Input: part model. Units: mm. Frame: model coordinates. Face numbers are marked on the shaded views. Give positions to 0.01 mm unless a question says otherwise; leave off trailing zeros. Order: outer loops, then holes, each group sorted by start corner. A loop starts at its lowest first (then second) coordinate and runs counter-clockwise, first axis right, second up. Notation, with made-up numbers: (54.25, 81) -> (76.25, 81) arc R29 cw to (76.25, 103) -> close; hole circle Ø1 at (38, 19). An arc over 180 degrees is marked (long way). Use a Markdown table: item, result. Add a question column.
Autodesk Inventor part; units mm, degrees
ref_plane "YZ Plane" through (0, 0, 0) normal (1, 0, 0) x (0, 1, 0)
ref_plane "XZ Plane" through (0, 0, 0) normal (0, 1, 0) x (-1, 0, 0)
ref_plane "XY Plane" through (0, 0, 0) normal (0, 0, 1) x (1, 0, 0)
sketch "Skizze2" plane through (0, 0, 0) normal (0, 0, 1) x (1, 0, 0)
  line L0 (-26.1954, 0) -> (26.1954, 0)
  line L1 (0, -30.2532) -> (0, 68.0422)
  line L2 (-18.5, 54) -> (-18.5, -6.7574)
  line L3 (-9.2574, -16) -> (9.2574, -16)
  line L4 (18.5, -6.7574) -> (18.5, 54)
  line L5 (18.5, 54) -> (11, 54)
  line L6 (11, 54) -> (11, 4.2426)
  line L7 (-11, 4.2426) -> (-11, 54)
  line L8 (-11, 54) -> (-18.5, 54)
  circle A0 centre (0, -10) radius 3.15
  circle A1 centre (-14.75, 43) radius 1.15
  circle A2 centre (-14.75, 30) radius 1.15
  circle A3 centre (-14.75, 17) radius 1.15
  circle A4 centre (-14.75, 3) radius 1.15
  circle A5 centre (14.75, 43) radius 1.15
  circle A6 centre (14.75, 30) radius 1.15
  circle A7 centre (14.75, 17) radius 1.15
  circle A8 centre (14.75, 3) radius 1.15
  line L9 (-17.6213, -8.8787) -> (-11.3787, -15.1213)
  line L10 (11.3787, -15.1213) -> (17.6213, -8.8787)
  arc A9 (-18.5, -6.7574) -> (-17.6213, -8.8787) centre (-15.5, -6.7574) ccw
  arc A10 (-11.3787, -15.1213) -> (-9.2574, -16) centre (-9.2574, -13) ccw
  arc A11 (9.2574, -16) -> (11.3787, -15.1213) centre (9.2574, -13) ccw
  line L11 (-11, 4.2426) -> (-11, 1.4853)
  line L12 (11, 4.2426) -> (11, 1.4853)
  line L13 (-6.7574, -2.7574) -> (6.7574, -2.7574)
  line L14 (-10.1213, -0.636) -> (-8.8787, -1.8787)
  line L15 (8.8787, -1.8787) -> (10.1213, -0.636)
  arc A12 (-11, 1.4853) -> (-10.1213, -0.636) centre (-8, 1.4853) ccw
  arc A13 (-8.8787, -1.8787) -> (-6.7574, -2.7574) centre (-6.7574, 0.2426) ccw
  arc A14 (6.7574, -2.7574) -> (8.8787, -1.8787) centre (6.7574, 0.2426) ccw
  arc A15 (10.1213, -0.636) -> (11, 1.4853) centre (8, 1.4853) ccw
  arc A16 (17.6213, -8.8787) -> (18.5, -6.7574) centre (15.5, -6.7574) ccw
  point P0 (0, 0)
  point P1 (-18.5, -16)
  point P2 (18.5, -16)
  point P3 (11, 0)
  point P4 (-11, 0)
  point P5 (-8, 0)
  point P6 (-11, 3)
  point P7 (8, 0)
  point P8 (11, 3)
  point P9 (-18.5, -8)
  point P10 (-10.5, -16)
  point P11 (10.5, -16)
  point P12 (18.5, -8)
  point P13 (-11, -2.7574)
  point P14 (11, -2.7574)
  point P15 (-11, 0.2426)
  point P16 (-8, -2.7574)
  point P17 (8, -2.7574)
  point P18 (11, 0.2426)
  dimension "d0" = 70
  dimension "d1" = 37
  dimension "d2" = 90
  dimension "d3" = 70
  dimension "d4" = 90
  dimension "d6" = 7.5
  dimension "d8" = 90
  dimension "d9" = 22
  dimension "d10" = 54
  dimension "d11" = 6.3
  dimension "d13" = 6
  dimension "d14" = 2.3
  dimension "d15" = 3.75
  dimension "d16" = 11
  dimension "d17" = 2.3
  dimension "d18" = 2.3
  dimension "d19" = 2.3
  dimension "d20" = 13
  dimension "d21" = 13
  dimension "d22" = 14
  dimension "d23" = 3.75
  dimension "d24" = 3.75
  dimension "d25" = 3.75
  dimension "d26" = 2.3
  dimension "d27" = 2.3
  dimension "d28" = 2.3
  dimension "d29" = 2.3
  dimension "d30" = 3.75
  dimension "d31" = 3
  dimension "d32" = 3
  dimension "d33" = 3
  dimension "d34" = 3
  dimension "d35" = 8
  dimension "d36" = 8
  dimension "d37" = 8
  dimension "d38" = 8
  dimension "d45" = 7
  dimension "d46" = 7
  dimension "d47" = 3
  dimension "d48" = 3
  dimension "d49" = 3
  dimension "d50" = 3
  dimension "d51" = 3
  dimension "d52" = 90
  dimension "d53" = 54
  dimension "d54" = 2.7574
  dimension "d55" = 11
  dimension "d56" = 8
  dimension "d57" = 8
  dimension "d58" = 3
extrude "Extrusion1" add sketch "Skizze2" along normal blind 4 contours L2 L8 L7 L11 A12 L0 | L0 A12 L14 A13 L13 L1 A0 L3 A10 L9 A9 L2 | A15 L12 L6 L5 L4 L0 | L0 L4 A16 L10 A11 L3 L1 A0 L13 A14 L15 A15
equation "\"d14\" = d29"
equation "\"d17\" = d28"
equation "\"d18\" = d28"
equation "\"d19\" = d29"
equation "\"d23\" = d24"
equation "\"d24\" = d25"
equation "\"d25\" = d15"
equation "\"d26\" = d29"
equation "\"d27\" = d28"
equation "\"d28\" = d29"
equation "\"d30\" = d15"
properties part number "Part1_new1" material "Aluminium 6061"
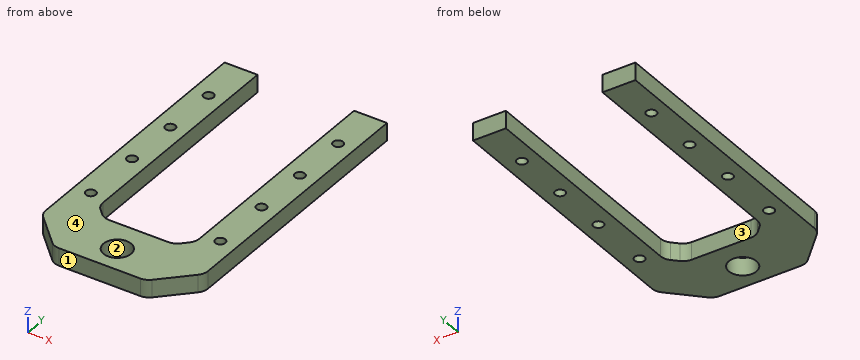
Q1. Section query B-B (x = -14.75). Return loops of the section in (y, z).
Q2. Section query D-D (y = 43). Return loops of the section in (x, z), plus the area to 3 significant figures.
Q3. Section query A-A (y = -10). Return loops of the section in (x, z), plus the area to 3 significant figures.
Q4. Draft query along Y for the marked faces 1, 2, 3 and 4. Return one class per face: +Y half, -Y half, draft (parallel to the pull), parting line (faces both ways), or undercut.
Q5. Section query C-C (x = 0). Return loops of the section in (y, z).
Q6. Ray query, line 1 (X direction, y = 25, z = 0.85); line 2 (Y direction, x = 14.75, z = 2.5); line 3 (X direction, y = 16.5, z = 0.6). Return the intervals inside material, ascending.
Solution:
| question | item | result |
|---|---|---|
| 1 | outline | (-11.75, 0) -> (1.85, 0) -> (1.85, 4) -> (-11.75, 4) -> close; (4.15, 0) -> (15.85, 0) -> (15.85, 4) -> (4.15, 4) -> close; (18.15, 0) -> (28.85, 0) -> (28.85, 4) -> (18.15, 4) -> close; (31.15, 0) -> (41.85, 0) -> (41.85, 4) -> (31.15, 4) -> close; (44.15, 0) -> (54, 0) -> (54, 4) -> (44.15, 4) -> close |
| 2 | outline | (-18.5, 0) -> (-15.9, 0) -> (-15.9, 4) -> (-18.5, 4) -> close; (-13.6, 0) -> (-11, 0) -> (-11, 4) -> (-13.6, 4) -> close; (11, 0) -> (13.6, 0) -> (13.6, 4) -> (11, 4) -> close; (15.9, 0) -> (18.5, 0) -> (18.5, 4) -> (15.9, 4) -> close |
| 2 | area | 41.6 mm² |
| 3 | outline | (-16.5, 0) -> (-3.15, 0) -> (-3.15, 4) -> (-16.5, 4) -> close; (3.15, 0) -> (16.5, 0) -> (16.5, 4) -> (3.15, 4) -> close |
| 3 | area | 107 mm² |
| 4 | face 1 | -Y half |
| 4 | face 2 | undercut |
| 4 | face 3 | +Y half |
| 4 | face 4 | draft |
| 5 | outline | (-16, 0) -> (-13.15, 0) -> (-13.15, 4) -> (-16, 4) -> close; (-6.85, 0) -> (-2.76, 0) -> (-2.76, 4) -> (-6.85, 4) -> close |
| 6 | line 1 | x = -18.5 to -11, 11 to 18.5 |
| 6 | line 2 | y = -11.75 to 1.85, 4.15 to 15.85, 18.15 to 28.85, 31.15 to 41.85, 44.15 to 54 |
| 6 | line 3 | x = -18.5 to -15.79, -13.71 to -11, 11 to 13.71, 15.79 to 18.5 |
